The listing builds one solid part. Answer for the finished solid, in the listing's coordinates (mm). A direction names the side the tool comes from. Give positions to 0.01 mm unless a question says otherwise; leave off trailing zeros. Order: outer loops, then holes, each group sorted by start corner. A loop starts at its lowest first (then second) coordinate and runs counter-clockwise, first axis right, second up. Notation, with made-up numbers: (-31.75, 64) - (-27.75, 64) arc R18 cw to (-27.75, 77) - close; hole circle Ø8 at (16, -29.75). An arc over 180 degrees is marked (long way). Write each question's results on one line, items separated by ' | '. Start each with the question number.
1. Determine the mould class of faces 4 (the face through (-1, 29, 9)), 5 (the face through (52.5, 0, 5)), 6 (the face through (-58, 15, 5)) for opening direction Y: released by +Y, released by -Y, zero draft, split by the parting line, or undercut.
2. Which of the six approach directions +Z, -Z, +X, -X, +Y, -Y give full straight-line access (tool end or side, diameter ignored) to faces 1 (the face through (57.25, -13.13, 5.99)), 2 (the face through (56.5, 0, 1)), 3 (the face through (-56.5, 0, 9))?
3. Section B-B (y = -2) is taken. Give the vertices of the cut face in (x, z), and give its area (3 significant figures).
4. Find the intervals of material crossed by L1, parallel to Z at x = 57.45, y = 13; L2, parallel to Y at x = -24.5, z = 1.5; L3, parallel to X at y = -20, z = 3, in increasing order.
5. Flat-ended cylindrical pins translate along their axes: pin 1 (0.8 mm diameter, centred on x = -57, y = -8.5, fed in from -Z); pin 2 (0.5 mm diameter, centred on x = -57, z = 6, fed in from -Y); pin 3 (3 mm diameter, centred on x = 55.5, z = 4, fed in from -Y). Find the tip coordinate at first contact, or state that the pin passes through.
6. Section A-A (y = 8) is taken. Give the vertices of the cut face in (x, z).
from build123d import *

# Parameters (mm, degrees)
F0_W       = 113
F0_H       = 58
F1_DEPTH   = 10
F2_R       = 5
F3_R       = 5
F4_R       = 5
F5_R       = 5
F6_W       = 1
F6_H       = 10
F11_DEPTH  = 1
F10_W      = 48
F10_H      = 6
F12_DEPTH  = 1
F7_W       = 103
F7_H       = 6
F13_DEPTH  = 1
F8_W       = 48
F8_H       = 6
F14_DEPTH  = 1
F9_W       = 103
F9_H       = 6
F15_DEPTH  = 1
F16_W      = 22
F16_H      = 4
F17_DEPTH  = 5
F18_R      = 1
F19_DEPTH  = 0.5
F19_FACE_R = 1
F20_DEPTH  = 0.5
F21_DEPTH  = 0.5
F22_R      = 1
F23_DEPTH  = 0.5
F24_W      = 5.293664
F24_H      = 2
F25_DEPTH  = 1.5
F26_W      = 7
F26_H      = 1.853713
F28_DEPTH  = 1.5
F31_DEPTH  = 0.5
F32_R      = 2.5
F33_DEPTH  = 5
F33_FACE_R = 2.5
F34_DEPTH  = 5


with BuildPart() as f1:
    # F0 (on Top) → F1 (new body)
    with BuildSketch(Plane.XY):
        Rectangle(F0_W, F0_H)
    extrude(amount=F1_DEPTH)

    # F2
    f2_edges = [f1.edges().sort_by_distance(p)[0] for p in [
        (56.5, 29, 5),
    ]]
    fillet(f2_edges, radius=F2_R)

    # F3
    f3_edges = [f1.edges().sort_by_distance(p)[0] for p in [
        (56.5, -29, 5),
    ]]
    fillet(f3_edges, radius=F3_R)

    # F4
    f4_edges = [f1.edges().sort_by_distance(p)[0] for p in [
        (-56.5, -29, 5),
    ]]
    fillet(f4_edges, radius=F4_R)

    # F5
    f5_edges = [f1.edges().sort_by_distance(p)[0] for p in [
        (-56.5, 29, 5),
    ]]
    fillet(f5_edges, radius=F5_R)

    # F6 (on face) → F11 (cut)
    with BuildSketch(Plane.XY.offset(10)):
        with Locations((-48, 1)):
            Rectangle(F6_W, F6_H)
    extrude(amount=-F11_DEPTH, mode=Mode.SUBTRACT)

    # F10 (on face) → F12 (join)
    with BuildSketch(Plane(origin=(-56.5, 0, 0), x_dir=(0, -1, 0), z_dir=(-1, 0, 0))):
        with Locations((0, 5)):
            Rectangle(F10_W, F10_H)
    extrude(amount=F12_DEPTH)

    # F7 (on face) → F13 (join)
    with BuildSketch(Plane(origin=(0, 29, 0), x_dir=(-1, 0, 0), z_dir=(0, 1, 0))):
        with Locations((0, 5)):
            Rectangle(F7_W, F7_H)
    extrude(amount=F13_DEPTH)

    # F8 (on face) → F14 (join)
    with BuildSketch(Plane.YZ.offset(56.5)):
        with Locations((0, 5)):
            Rectangle(F8_W, F8_H)
    extrude(amount=F14_DEPTH)

    # F9 (on face) → F15 (join)
    with BuildSketch(Plane.XZ.offset(29)):
        with Locations((0, 5)):
            Rectangle(F9_W, F9_H)
    extrude(amount=F15_DEPTH)

    # F16 (on face) → F17 (cut)
    with BuildSketch(Plane.YZ.offset(57.5)):
        with Locations((0, 5)):
            Rectangle(F16_W, F16_H)
    extrude(amount=-F17_DEPTH, mode=Mode.SUBTRACT)

    # F18 (on face) → F19 (join)
    with BuildSketch(Plane.YZ.offset(57.5)):
        with Locations((13, 5)):
            Circle(F18_R)
    extrude(amount=F19_DEPTH)

    # F19_face (on face) → F20 (cut)
    with BuildSketch(Plane(origin=(58, 13, 5), x_dir=(0, 1, 0), z_dir=(1, 0, 0))):
        Circle(F19_FACE_R)
    extrude(amount=-F20_DEPTH, mode=Mode.SUBTRACT)

    # F18 (on face) → F21 (cut)
    with BuildSketch(Plane.YZ.offset(57.5)):
        with Locations((13, 5)):
            Circle(F18_R)
    extrude(amount=-F21_DEPTH, mode=Mode.SUBTRACT)

    # F22 (on face) → F23 (cut)
    with BuildSketch(Plane.YZ.offset(57.5)):
        with Locations((-13, 5)):
            Circle(F22_R)
    extrude(amount=-F23_DEPTH, mode=Mode.SUBTRACT)

    # F24 (on face) → F25 (cut)
    with BuildSketch(Plane.YZ.offset(57.5)):
        with Locations((17.646832, 5)):
            Rectangle(F24_W, F24_H)
    extrude(amount=-F25_DEPTH, mode=Mode.SUBTRACT)

    # F26 (on face) → F28 (cut)
    with BuildSketch(Plane.YZ.offset(57.5)):
        with Locations((-18.5, 5.073144)):
            Rectangle(F26_W, F26_H)
    extrude(amount=-F28_DEPTH, mode=Mode.SUBTRACT)

    # F30 (on face) → F31 (join)
    with BuildSketch(Plane(origin=(-57.5, 0, 0), x_dir=(0, -1, 0), z_dir=(-1, 0, 0))):
        with BuildLine():
            Line((-19, 4), (-11, 4))
            ThreePointArc((-11, 4), (-10.292893, 4.292893), (-10, 5))
            ThreePointArc((-10, 5), (-10.292893, 5.707107), (-11, 6))
            Line((-11, 6), (-19, 6))
            ThreePointArc((-19, 6), (-19.707107, 5.707107), (-20, 5))
            ThreePointArc((-20, 5), (-19.707107, 4.292893), (-19, 4))
        make_face()
    extrude(amount=F31_DEPTH)

    # F32 (on face) → F33 (join)
    with BuildSketch(Plane(origin=(-57.5, 0, 0), x_dir=(0, -1, 0), z_dir=(-1, 0, 0))):
        with Locations((16.500002, 5.005926)):
            Circle(F32_R)
    extrude(amount=F33_DEPTH)

    # F33_face (on face) → F34 (cut)
    with BuildSketch(Plane(origin=(-62.5, -16.500002, 5.005926), x_dir=(0, -1, 0), z_dir=(-1, 0, 0))):
        Circle(F33_FACE_R)
    extrude(amount=-F34_DEPTH, mode=Mode.SUBTRACT)


solid = f1.part
Reported:
1) face 4: released by +Y | face 5: undercut | face 6: zero draft
2) face 1: +X | face 2: -Z, +X, +Y, -Y | face 3: +Z, -X, +Y, -Y
3) outline: (-57.5, 2) - (-56.5, 2) - (-56.5, 0) - (56.5, 0) - (56.5, 2) - (57.5, 2) - (57.5, 3) - (52.5, 3) - (52.5, 7) - (57.5, 7) - (57.5, 8) - (56.5, 8) - (56.5, 10) - (-47.5, 10) - (-47.5, 9) - (-48.5, 9) - (-48.5, 10) - (-56.5, 10) - (-56.5, 8) - (-57.5, 8) - close | area: 1,120 mm²
4) L1: 2 to 4, 6 to 8 | L2: -29 to 29 | L3: -57.5 to 57.5
5) pin 1: z = 2 | pin 2: y = -24 | pin 3: y = -28.33
6) outline: (-57.5, 2) - (-56.5, 2) - (-56.5, 0) - (56.5, 0) - (56.5, 2) - (57.5, 2) - (57.5, 3) - (52.5, 3) - (52.5, 7) - (57.5, 7) - (57.5, 8) - (56.5, 8) - (56.5, 10) - (-56.5, 10) - (-56.5, 8) - (-57.5, 8) - close
